Here's how the part is built. I have some questions about the finished solid (model axes, mm). A direction names the side the tool comes from. Coordinates: 2 decimals unless noted, no trailing zeros. Loops run counter-clockwise (first coordinate to the right, second up) from the corner with the lowest first, then second, coordinate; pieces in that order, holes last. Notation, with made-up numbers: M 7,82.25 L 40,82.25 A29 cw 40,106.25 Z; hole C -36.5,66.25 d9. An arc over 180 degrees is marked long. Use CSV: the item, a comma, the result in double quotes. Start each with the question number.
Q1. Please list where these lines run through material, in increasing order: probe 1 along Z at (x, y) = (19.05, -9) (3 decimals); probe 2 along Y at (x, z) = (14.5, -1.5); probe 3 along X at (y, z) = (-3.5, -1.5). Write a range as [from, to].
Q2. If we section it at C-C (z = -1): Please give me the cut outline in (x, y).
Q3. If we mould it in two halves opening along Y, with no side actions, what happens to faces 1 (the cylindrical face through (12.458, 3.706, 1.565)), 2 (the cylindrical face through (0.955, 11.11, 1.61)), 3 (the flat face through (20, -13.385, -4))? For each: +Y half, -Y half, draft (parallel to the pull), parting line (faces both ways), or undercut.
Q4. If we section it at D-D (x = 4.5): Please give me the cut outline in (y, z) (3 decimals), and give its area (3 significant figures).
Q5. For pin 1 Ø5 at (y, z) = (8, 1.5) entering from +X; pin 2 Ø3 at (y, z) = (1.5, -3) entering from +X; pin 3 Ø5 at (x, z) = (17, -3.5) entering from -Y, each with a flat end and sliding along its axis, tell me the tip position at first contact or that it passes through.
Q6. Which directions (+Z, -Z, +X, -X, +Y, -Y) give clear straight access to the entire face, cutting with the end or side of a thin tool? Please do faces 4 (the flat face through (20, -0.685, -4)), 5 (the flat face through (19.05, -20, 2)), 6 (the flat face through (19.05, 6, 2)).
Q7. If we section it at B-B (z = 2.5): Please give me the cut outline in (x, y) (3 decimals).
Autodesk Inventor part; units mm, degrees
ref_plane "Work Plane1" through (3.175, -7.0346, 3.175) normal (0, 1, 0) x (1, 0, 0)
ref_plane "YZ Plane" through (0, 0, 0) normal (1, 0, 0) x (0, 1, 0)
ref_plane "XZ Plane" through (0, 0, 0) normal (0, 1, 0) x (-1, 0, 0)
sketch "Sketch1" plane through (0, 0, 0) normal (0, 0, 1) x (1, 0, 0)
  line L0 (0, 12.0154) -> (19.05, 12.0154)
  line L1 (19.05, 12.0154) -> (19.05, -26.0846)
  line L2 (19.05, -26.0846) -> (0, -26.0846)
  line L3 (0, -26.0846) -> (0, 12.0154)
  circle A0 centre (9.525, 2.4904) radius 3.175
  circle A1 centre (9.525, -16.5596) radius 3.175
  point P0 (0, 0)
  dimension "d0" = 19.05
  dimension "d1" = 38.1
  dimension "d2" = 6.35
  dimension "d3" = 6.35
  dimension "d4" = 19.05
  dimension "d5" = 9.525
  dimension "d6" = 9.525
extrude "Extrusion1" add sketch "Sketch1" along normal blind 3.175
fillet "Fillet1" radius 3.175 2 edges at (0, 12.0154, 1.5875) (0, -26.0846, 1.5875)
ref_plane "Work Plane1" through (3.175, -7.0346, 3.175) normal (0, 1, 0) x (1, 0, 0)
sketch "Sketch3" plane through (3.175, -7.0346, 3.175) normal (0, 1, 0) x (1, 0, 0)
  circle A0 centre (15.875, 4.7625) radius 4.7625
  line L0 (0, 3.175) -> (15.875, 3.175)
  line L1 (15.875, 0) -> (0, 0)
  point P0 (-3.175, 3.175)
  dimension "d21" = 9.525
extrude "Extrusion4" add sketch "Sketch3" along normal mid plane 12.7
sketch "Sketch6" plane through (19.05, 12.0154, 3.175) normal (0, 1, 0) x (1, 0, 0)
  circle A0 centre (0, 4.7625) radius 2.3813
  arc A1 (0, 0) -> (-4.4901, 3.175) centre (0, 4.7625) ccw
  point P0 (-19.05, 3.175)
  point P1 (-4.4901, 0)
  point P2 (0, 3.175)
  dimension "d18" = 4.7625
extrude "Extrusion5" cut sketch "Sketch6" against normal blind 38.1
sketch "Sketch8" plane through (0, 0, 0) normal (0, 1, 0) x (-1, 0, 0)
  arc A0 (-19.05, 0.7937) -> (-17.2751, 0) centre (-19.05, -1.5875) ccw
  line L0 (-14.5599, 0) -> (-17.2751, 0)
  arc A1 (-19.05, 3.175) -> (-14.5599, 0) centre (-19.05, -1.5875) ccw
  line L1 (-19.05, 0.7937) -> (-19.05, 3.175)
  line L2 (-3.175, 3.175) -> (0, 3.175)
  line L3 (0, 3.175) -> (0, 0)
  line L4 (0, 0) -> (-3.175, 0)
  line L5 (-3.175, 0) -> (-3.175, 3.175)
  line L6 (0, 0) -> (-14.2875, 0)
  line L7 (-14.2875, 0) -> (-14.2875, -6.4324)
  line L8 (-14.2875, -6.4324) -> (0, -6.4324)
  line L9 (0, -6.4324) -> (0, 0)
  dimension "d22" = 14.2875
equation "\"d3\" = d2"
equation "\"d4\" = 0.5 * d1"
equation "\"d5\" = 0.25 * d1"
equation "\"d6\" = 0.5 * d0"
properties part number "hinge right" material "Brass, Soft Yellow"
Results below:
1,probe 1,"[-6.35, -3.969], [0.794, 3.175]"
1,probe 2,"[-13.38, -0.68]"
1,probe 3,"[14.29, 16.67], [21.43, 23.81]"
2,outline,"M 14.32,-13.38 L 16.74,-13.38 L 16.74,-0.68 L 14.32,-0.68 Z; M 21.36,-13.38 L 23.78,-13.38 L 23.78,-0.68 L 21.36,-0.68 Z"
3,face 1,"undercut"
3,face 2,"+Y half"
3,face 3,"-Y half"
4,outline,"M -26.085,0 L 12.015,0 L 12.015,3.175 L -26.085,3.175 Z"
4,area,"121 mm^2"
5,pin 1,"x = 19.05"
5,pin 2,"through"
5,pin 3,"y = -13.38"
6,face 4,"-Z, +X, +Y"
6,face 5,"+Z, -Z, +X, -Y"
6,face 6,"+Z, -Z, +X, +Y"
7,outline,"M 0,-22.91 A3.175 ccw 3.175,-26.085 L 19.05,-26.085 L 19.05,-13.385 L 21.494,-13.385 L 21.494,-0.685 L 19.05,-0.685 L 19.05,12.015 L 3.175,12.015 A3.175 ccw 0,8.84 Z; hole C 9.525,-16.56 d6.35; hole C 9.525,2.49 d6.35"
